CAD build for the part. Positions are in the model's coordinates, mm. Coordinates: 2 decimals unless noted, no trailing zeros. Loops run counter-clockwise (first coordinate to the right, second up) from the corner with the lowest first, then second, coordinate; pieces in that order, holes last. Notation, with made-up numbers: (8.25, 19) -> (52.25, 19) arc R6 ccw to (52.25, 29) -> close; hole circle Ø10 at (-4, 7.25). An arc over 180 degrees is marked (long way). Return JSON: item names as keys, results as strings. Group by question number.
(1) Saw through at B-B on y = 0.1. Write the cut outline in (x, z), then the cut area to 3 significant figures.
(2) Saw through at A-A on z = 5.75. Write the cut outline in (x, y).
(3) Flat gauge pin, fed straight in: pin 1 Ø4 at (x, z) = (2, 2) entering from +Y. Where does the tip first touch, or does it go through?
(4) Probe L1, parallel to X at y = -0.25, z = 3.75; L2, parallel to Z at x = 2.5, y = 0.45; L3, parallel to X at y = 0.9, z = 0.25. List the from-to ranges inside material, lowest first.
(5) Saw through at D-D on z = -0.5. Write the cut outline in (x, y), then the cut area to 3 significant figures.
(6) Saw through at C-C on x = -10. Write the cut outline in (y, z), then the cut area to 3 significant figures.
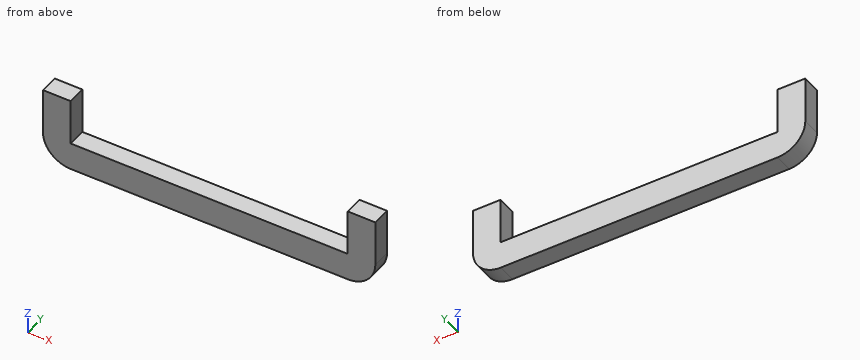
```python
from build123d import *

# Parameters (mm, degrees)
SKETCH1_W           = 36
SKETCH1_H           = 3
SKETCH1_W_2         = 3
SKETCH1_H_2         = 5
BOSS_EXTRUDE1_DEPTH = 1
FILLET1_R           = 3


with BuildPart() as part:
    # Sketch1 → Boss-Extrude1 (new, symmetric)
    with BuildSketch(Plane(origin=(0, 0, 0), x_dir=(1, 0, 0), z_dir=(0, 1, 0))):
        Rectangle(SKETCH1_W, SKETCH1_H)
        with Locations((-16.5, -4)):
            Rectangle(SKETCH1_W_2, SKETCH1_H_2)
        with Locations((16.5, -4)):
            Rectangle(SKETCH1_W_2, SKETCH1_H_2)
    extrude(amount=BOSS_EXTRUDE1_DEPTH, both=True)

    # Fillet1
    fillet1_edges = [part.edges().sort_by_distance(p)[0] for p in [
        (-18, 0, -1.5),
        (18, 0, -1.5),
    ]]
    fillet(fillet1_edges, radius=FILLET1_R)


solid = part.part
```
Geometry results:
{
 "1": {"outline": "(-18, 1.5) arc R3 ccw to (-15, -1.5) -> (15, -1.5) arc R3 ccw to (18, 1.5) -> (18, 6.5) -> (15, 6.5) -> (15, 1.5) -> (-15, 1.5) -> (-15, 6.5) -> (-18, 6.5) -> close", "area": "134 mm²"},
 "2": {"outline": "(-18, -1) -> (-15, -1) -> (-15, 1) -> (-18, 1) -> close; (15, -1) -> (18, -1) -> (18, 1) -> (15, 1) -> close"},
 "3": {"pin 1": "y = 1"},
 "4": {"L1": "-18 to -15, 15 to 18", "L2": "-1.5 to 1.5", "L3": "-17.73 to 17.73"},
 "5": {"outline": "(-17.24, -1) -> (17.24, -1) -> (17.24, 1) -> (-17.24, 1) -> close", "area": "68.9 mm²"},
 "6": {"outline": "(-1, -1.5) -> (1, -1.5) -> (1, 1.5) -> (-1, 1.5) -> close", "area": "6.00 mm²"}
}
